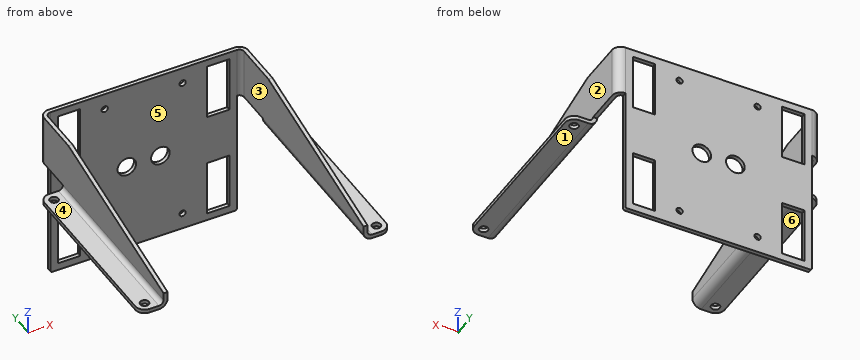
from build123d import *

# Parameters (mm, degrees)
F1_DEPTH  = 21.70684
F2_W      = 1.70942
F2_H      = 79.1155667
F3_DEPTH  = 3.69316
F4_W      = 9.92124
F4_H      = 1.70942
F5_DEPTH  = 79.1155667
F6_W      = 79.3829248
F6_H      = 1.70942
F7_DEPTH  = 54.49316
F8_W      = 9.5329248
F8_H      = 24
F8_R      = 1.35255
F8_R_2    = 3.96875
F9_DEPTH  = 1.70942
F10_R     = 0.762
F11_R     = 3.96875
F12_R     = 3.69316
F13_R     = 1.98374
F15_DEPTH = 86.7692448
F16_R     = 1.8288
F17_DEPTH = 1.70942


with BuildPart() as f1:
    # F0 (on Top) → F1 (new body)
    with BuildSketch(Plane.XY):
        Polygon((-1.70942, -95.9058534), (0, -95.9058534), (0, 0), (83.3504048, 0), (83.3504048, -95.9058534), (85.0598248, -95.9058534), (85.0598248, 1.70942), (-1.70942, 1.70942), align=None)
    extrude(amount=F1_DEPTH)

    # F2 (on face) → F3 (join)
    with BuildSketch(Plane(origin=(0, 0, 0), x_dir=(1, 0, 0), z_dir=(0, 0, -1))):
        with Locations((-0.85471, 56.34807005)):
            Rectangle(F2_W, F2_H)
        with Locations((84.2051148, 56.34807005)):
            Rectangle(F2_W, F2_H)
    extrude(amount=F3_DEPTH)

    # F4 (on face) → F5 (join, through all)
    with BuildSketch(Plane.XZ.offset(95.9058534)):
        with Locations((90.0204448, -2.83845)):
            Rectangle(F4_W, F4_H)
        with Locations((-6.67004, -2.83845)):
            Rectangle(F4_W, F4_H)
    extrude(amount=-F5_DEPTH)

    # F6 (on face) → F7 (join)
    with BuildSketch(Plane(origin=(0, 0, 0), x_dir=(1, 0, 0), z_dir=(0, 0, -1))):
        with Locations((41.6752024, -0.85471)):
            Rectangle(F6_W, F6_H)
    extrude(amount=F7_DEPTH)

    # F8 (on face) → F9 (cut, through all)
    with BuildSketch(Plane(origin=(0, 1.70942, 0), x_dir=(-1, 0, 0), z_dir=(0, 1, 0))):
        with Locations((-9.9252024, -39.31816)):
            Rectangle(F8_W, F8_H)
        with Locations((-9.9252024, 6.53184)):
            Rectangle(F8_W, F8_H)
        with Locations((-73.4252024, 6.53184)):
            Rectangle(F8_W, F8_H)
        with Locations((-73.4252024, -39.31816)):
            Rectangle(F8_W, F8_H)
        with Locations((-25.0871228, -47.34941)):
            Circle(F8_R)
        with Locations((-58.263282, -47.34941)):
            Circle(F8_R)
        with Locations((-58.263282, 14.56309)):
            Circle(F8_R)
        with Locations((-25.0871228, 14.56309)):
            Circle(F8_R)
        with Locations((-48.8189524, -16.39316)):
            Circle(F8_R_2)
        with Locations((-34.5314524, -16.39316)):
            Circle(F8_R_2)
    extrude(amount=-F9_DEPTH, mode=Mode.SUBTRACT)

    # F10
    f10_edges = [f1.edges().sort_by_distance(p)[0] for p in [
        (1.98374, 0.85471, -54.49316),
        (81.366665, 0.85471, -54.49316),
    ]]
    fillet(f10_edges, radius=F10_R)

    # F11
    f11_edges = [f1.edges().sort_by_distance(p)[0] for p in [
        (94.981065, -95.905853, -2.83845),
        (-11.63066, -16.790287, -2.83845),
        (-11.63066, -95.905853, -2.83845),
        (94.981065, -16.790287, -2.83845),
    ]]
    fillet(f11_edges, radius=F11_R)

    # F12
    f12_edges = [f1.edges().sort_by_distance(p)[0] for p in [
        (0, -56.34807, -3.69316),
        (-1.70942, 1.70942, 10.85342),
        (85.059825, 1.70942, 10.85342),
        (83.350405, -56.34807, -3.69316),
    ]]
    fillet(f12_edges, radius=F12_R)

    # F13
    f13_edges = [f1.edges().sort_by_distance(p)[0] for p in [
        (83.350405, 0, 10.85342),
        (0, 0, 10.85342),
        (85.059825, -56.34807, -1.98374),
        (-1.70942, -56.34807, -1.98374),
    ]]
    fillet(f13_edges, radius=F13_R)

    # F14 (on face) → F15 (cut, through all)
    with BuildSketch(Plane(origin=(-1.70942, 0, 0), x_dir=(0, -1, 0), z_dir=(-1, 0, 0))):
        Polygon((95.9058534, 21.70684), (21.03374, 21.70684), (95.9058534, 3.175), align=None)
    extrude(amount=-F15_DEPTH, mode=Mode.SUBTRACT)

    # F16 (on face) → F17 (cut, through all)
    with BuildSketch(Plane(origin=(0, 0, -3.69316), x_dir=(1, 0, 0), z_dir=(0, 0, -1))):
        with Locations((-7.66191, 91.9371034)):
            Circle(F16_R)
        with Locations((-7.66191, 20.7590367)):
            Circle(F16_R)
        with Locations((91.0123148, 91.9371034)):
            Circle(F16_R)
        with Locations((91.0123148, 20.7590367)):
            Circle(F16_R)
    extrude(amount=-F17_DEPTH, mode=Mode.SUBTRACT)


solid = f1.part
The model under review builds one solid part; all positions refer to its coordinate system, in mm. Face numbers are marked on the shaded views. A direction names the side the tool comes from. Round coordinates to 2 decimals unless told otherwise and drop trailing zeros. Loops run counter-clockwise (first coordinate to the right, second up) from the corner with the lowest first, then second, coordinate; pieces in that order, holes last. Notation, with made-up numbers: (76, 36) -> (96, 36) arc R27 ccw to (96, 53) -> close; hole circle Ø2 at (49.25, -22.75). An arc over 180 degrees is marked (long way). Write item = value, one per line. Start each with the question number.
Item 1: To check wall thickness, follow L1, parallel to X at y = -48, z = 5; L2, parallel to Y at x = 50.5, z = -33; L3, parallel to X at y = -24.5, z = -1.5 (3 decimals). State the ranges of each line that lie inside material, in increasing order.
Item 2: Take a section at D-D on x = 33. Give the boundary of the cut face in (y, z), plus the area to 3 significant figures.
Item 3: Mouldability with a two-part tool opening along X and no side actions: class the marked faces 1, 2 and 3 as released by +X, released by -X, zero draft, split by the parting line, or undercut.
Item 4: Insertion check: pin 1 (1.1 mm diameter, centred on x = 83, y = -10, fed in from -Z); pin 2 (11 mm diameter, centred on y = -28, z = 16, fed in from -X); pin 3 (4 mm diameter, centred on x = 15, z = 2, fed in from -Y). Each pin has a flat end and moves straight along its axis. Give the tip position at first contact, or say it passes through.
Item 5: For the marked faces 4, 5 and 6, list the 3-axis set-ups (+Z, -Z, +X, -X, +Y, -Y) from which the entire face can be reached by the end or side of a thin tool; tool diameter is ignored.
Item 6: Take a section at B-B on y = -14.5. Give the boundary of the cut face in (x, z), plus the area to 3 significant figures.
Item 7: Take a section at C-C on x = 10. Give the boundary of the cut face in (y, z).
Item 8: Take a section at A-A on z = -31. Give the boundary of the cut face in (x, y), plus the area to 3 significant figures.
Result:
q1.L1 = -1.71 to 0, 83.35 to 85.06
q1.L2 = 0 to 1.71
q1.L3 = -2.395 to -0.318, 83.669 to 85.745
q2.outline = (0, -54.49) -> (1.71, -54.49) -> (1.71, -20.05) -> (0, -20.05) -> close; (0, -12.73) -> (1.71, -12.73) -> (1.71, 21.71) -> (0, 21.71) -> close
q2.area = 118 mm²
q3.face_1 = zero draft
q3.face_2 = released by +X
q3.face_3 = undercut
q4.pin_1 = 0
q4.pin_2 = -1.71
q4.pin_3 = 0
q5.face_4 = +Z, -X, +Y, -Y
q5.face_5 = +Z, -Z, -Y
q5.face_6 = -Z, +X, -X, +Y, -Y
q6.outline = (-1.71, 0) -> (0, 0) -> (0, 21.71) -> (-1.71, 21.71) -> close; (83.35, 0) -> (85.06, 0) -> (85.06, 21.71) -> (83.35, 21.71) -> close
q6.area = 74.2 mm²
q7.outline = (0, -54.49) -> (1.71, -54.49) -> (1.71, -51.32) -> (0, -51.32) -> close; (0, -27.32) -> (1.71, -27.32) -> (1.71, -5.47) -> (0, -5.47) -> close; (0, 18.53) -> (1.71, 18.53) -> (1.71, 21.71) -> (0, 21.71) -> close
q8.outline = (1.98, 0) -> (5.16, 0) -> (5.16, 1.71) -> (1.98, 1.71) -> close; (14.69, 0) -> (68.66, 0) -> (68.66, 1.71) -> (14.69, 1.71) -> close; (78.19, 0) -> (81.37, 0) -> (81.37, 1.71) -> (78.19, 1.71) -> close
q8.area = 103 mm²
